```python
from build123d import *

# Parameters (mm, degrees)
F1_DEPTH = 30
F2_W     = 15
F2_H     = 40
F3_DEPTH = 23
F4_R     = 5
F5_DEPTH = 15
F6_R     = 9
F7_DEPTH = 27


with BuildPart() as f1:
    # F0 (on Front) → F1 (new body, symmetric)
    with BuildSketch(Plane.XZ):
        Polygon((-25, 35), (-40, 35), (-40, -15), (0, -15), (0, 0), (40, 0), (40, 35), (25, 35), (25, 12), (-25, 12), align=None)
    extrude(amount=F1_DEPTH, both=True)

    # F2 (on face) → F3 (cut, through all)
    with BuildSketch(Plane.XY.offset(35)):
        with Locations((32.5, 0)):
            Rectangle(F2_W, F2_H)
    extrude(amount=-F3_DEPTH, mode=Mode.SUBTRACT)

    # F4 (on face) → F5 (cut, through all)
    with BuildSketch(Plane.YZ.offset(-25)):
        with Locations((-15, 22)):
            Circle(F4_R)
        with Locations((15, 22)):
            Circle(F4_R)
    extrude(amount=-F5_DEPTH, mode=Mode.SUBTRACT)

    # F6 (on face) → F7 (cut, through all)
    with BuildSketch(Plane.XY.offset(12)):
        with Locations((-5, 0)):
            Circle(F6_R)
        with Locations((15, 0)):
            Circle(F6_R)
    extrude(amount=-F7_DEPTH, mode=Mode.SUBTRACT)


solid = f1.part
```
CAD build for the part. Positions are in the model's coordinates, mm. A direction names the side the tool comes from. Round coordinates to 2 decimals unless told otherwise and drop trailing zeros. Order: outer loops, then holes, each group sorted by start corner. A loop starts at its lowest first (then second) coordinate and runs counter-clockwise, first axis right, second up. Notation, with made-up numbers: (89, 9) -> (119, 9) arc R20 cw to (119, 16) -> close; hole circle Ø4 at (45.25, -29). An arc over 180 degrees is marked (long way). Write item = value, one per line.
(1) Cut at D-D (y = -15). Write the cut outline in (x, z), plus the area to 4 significant figures.
Answers follow:
outline = (-40, -15) -> (0, -15) -> (0, 0) -> (40, 0) -> (40, 12) -> (-25, 12) -> (-25, 17) -> (-40, 17) -> close; (-40, 27) -> (-25, 27) -> (-25, 35) -> (-40, 35) -> close
area = 1,755 mm²
(2) Cut at A-A (y = 0). Write the cut outline in (x, z), plus the area to 3 significant figures.
Answers follow:
outline = (-40, -15) -> (-14, -15) -> (-14, 12) -> (-25, 12) -> (-25, 35) -> (-40, 35) -> close; (4, 0) -> (6, 0) -> (6, 12) -> (4, 12) -> close; (24, 0) -> (40, 0) -> (40, 12) -> (24, 12) -> close
area = 1,260 mm²
(3) Flat gauge pins, fed straight in: P1, Ø23.5, axis at x = -5, y = 0, coming from the +Z side; P2, Ø7, axis at y = -10, z = 26, coming from the +X side; P3, Ø4.5, axis at y = -20.5, z = -4, coming from the +X side. Where does each tip first touch, or does it go through?
Answers follow:
P1 = 12
P2 = -25
P3 = 0
(4) Cut at B-B (x = 15). Write the cut outline in (y, z).
Answers follow:
outline = (-30, 0) -> (-9, 0) -> (-9, 12) -> (-30, 12) -> close; (9, 0) -> (30, 0) -> (30, 12) -> (9, 12) -> close
(5) Pull direction Y, two halves, no side cores. Call faces 6 (the cylindrical face through (-32.395, 17.307, 17.564)), 7 (the flat face through (25, -25, 24)), 8 (the flat face through (-9, -30, 10)): +Y half, -Y half, draft (parallel to the pull), parting line (faces both ways), or undercut.
Answers follow:
face_6 = undercut
face_7 = draft
face_8 = -Y half
(6) Cut at C-C (z = 22). Write the cut outline in (x, y), plus the area to 3 significant figures.
Answers follow:
outline = (-40, -30) -> (-25, -30) -> (-25, -20) -> (-40, -20) -> close; (-40, -10) -> (-25, -10) -> (-25, 10) -> (-40, 10) -> close; (-40, 20) -> (-25, 20) -> (-25, 30) -> (-40, 30) -> close; (25, -30) -> (40, -30) -> (40, -20) -> (25, -20) -> close; (25, 20) -> (40, 20) -> (40, 30) -> (25, 30) -> close
area = 900 mm²
(7) 3-axis set-ups, long thin cutter, end or side, ignore diameter. For faces 1 (the flat face through (25, 25, 24)), 2 (the flat face through (0, 19, -8)), 3 (the flat face through (32, 20, 24)), 4 (the flat face through (40, 0, 9)), 5 (the flat face through (-20, 0, -15)): which of +Z, -Z, +X, -X, +Y, -Y reach the whole face in a straight line?
Answers follow:
face_1 = +Z, +Y, -Y
face_2 = -Z, +X, +Y, -Y
face_3 = +Z, +X
face_4 = +Z, -Z, +X, +Y, -Y
face_5 = -Z, +X, -X, +Y, -Y
(8) Drill centre lines: L1, parallel to Y at x = 15, z = 7; L2, parallel to Z at x = -28, y = -15; L3, parallel to Y at x = 30, z = 29. Where is each one in solid material? Low to high.
Answers follow:
L1 = -30 to -9, 9 to 30
L2 = -15 to 17, 27 to 35
L3 = -30 to -20, 20 to 30
